from build123d import *

# Parameters (mm, degrees)
EXTRUDE_4_DEPTH     = 45
SKETCH_2_R          = 2.5
CUT_EXTRUDE_1_DEPTH = 85.798913103


with BuildPart() as part:
    # 草图1 → 凸台-拉伸4 (new body)
    with BuildSketch(Plane.XY):
        with BuildLine():
            ThreePointArc((11.999755772, 64.190702015), (7.19287537, 69.699227744), (0.441332655, 66.894477154))
            Line((0.441332655, 66.894477154), (-16.87917542, 36.894477154))
            Line((-16.87917542, 36.894477154), (-16.87917542, -3.105522846))
            Line((-16.87917542, -3.105522846), (-5.332170037, -23.105522846))
            Line((-5.332170037, -23.105522846), (9.992741519, -33.105522846))
            Line((9.992741519, -33.105522846), (11.999755772, -30.029791253))
            Line((11.999755772, -30.029791253), (-6.87917542, -3.105522846))
            Line((-6.87917542, -3.105522846), (-6.87917542, 14.190702015))
            Line((-6.87917542, 14.190702015), (-6.87917542, 24.190702015))
            Line((-6.87917542, 24.190702015), (10.114332844, 34.190702015))
            Line((10.114332844, 34.190702015), (11.999755772, 64.190702015))
        make_face()
    extrude(amount=EXTRUDE_4_DEPTH)

    # 草图2 → 切除-拉伸1 (cut, through all)
    with BuildSketch(Plane.XY):
        with Locations(Location((5.784422652, 63.881230161, 0), (0, 0, 180))):
            Circle(SKETCH_2_R)
    extrude(amount=CUT_EXTRUDE_1_DEPTH, mode=Mode.SUBTRACT)


solid = part.part
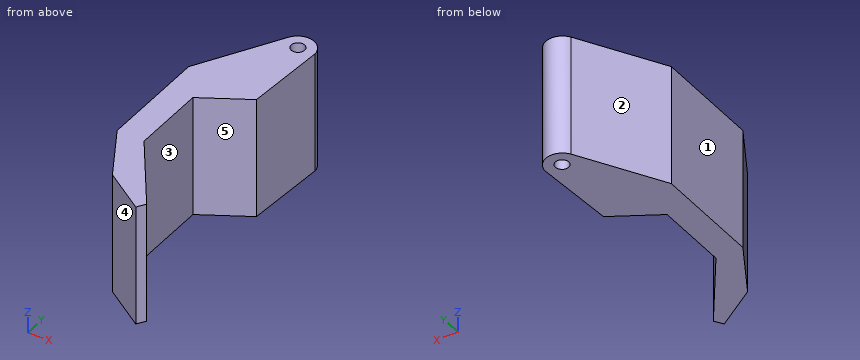
Can you work these out from the model? Positions are in its coordinate system, mm. Face numbers are marked on the shaded views. A direction names the side the tool comes from. Round coordinates to 2 decimals unless told otherwise and drop trailing zeros. Loops run counter-clockwise (first coordinate to the right, second up) from the corner with the lowest first, then second, coordinate; pieces in that order, holes last. Notation, with made-up numbers: (54.25, -5.5) - (70.25, -5.5) arc R21 cw to (70.25, 11.5) - close; hole circle Ø8 at (82.25, 22). An arc over 180 degrees is marked (long way). Use CSV: the item, a comma, the result in double quotes. Start each with the question number.
1) If we section it at C-C on x = -4: Write out the boundary of the cut face in (y, z).
2) For pin 1 Ø1 at (x, z) = (-5, 27.5) entering from +Y; pin 2 Ø4.5 at (x, y) = (5.78, 63.88) entering from +Z; pin 3 Ø12 at (x, z) = (1.5, 23.5) entering from -Y; pin 4 Ø5 at (x, z) = (-3.5, 29) entering from +Y, each with a flat end and sliding along its axis, tell me the tip position at first contact or that it passes through.
3) If we section it at B-B on z = 4.5: Write out the boundary of the cut face in (x, y), plus the area to 3 significant figures.
4) If we section it at A-A on x = 5.75: Write out the boundary of the cut face in (y, z).
5) For the marked faces 4 and 5, which set-ups out of +Z, -Z, +X, -X, +Y, -Y let a thin tool reach every point of the face, with its end or its side?
6) Please list where these lines run through material, in increasing order: probe 1 along Y at (x, z) = (6.5, 32); probe 2 along X at (y, z) = (3, 6); probe 3 along X at (y, z) = (63.5, 3). Write a range as [from, to].
7) If we section it at D-D on y = 17: Write out the boundary of the cut face in (x, z), plus the area to 3 significant figures.
8) We'd pull the mould along Y, two halves only. Please class the marked faces 1, 2 and 3: released by +Y, released by -Y, zero draft, split by the parting line, or undercut.
Geometry results:
1,outline,"(-23.97, 0) - (-7.21, 0) - (-7.21, 45) - (-23.97, 45) - close; (25.88, 0) - (59.2, 0) - (59.2, 45) - (25.88, 45) - close"
2,pin 1,"stops at y = 58.34"
2,pin 2,"passes through"
2,pin 3,"stops at y = -31.48"
2,pin 4,"stops at y = 64.4"
3,outline,"(-16.88, -3.11) - (-5.33, -23.11) - (9.99, -33.11) - (12, -30.03) - (-6.88, -3.11) - (-6.88, 24.19) - (10.11, 34.19) - (12, 64.19) arc R6.26 ccw to (0.44, 66.89) - (-16.88, 36.89) - close; hole circle Ø5 at (5.78, 63.88)"
3,area,"1,420 mm2"
4,outline,"(-30.34, 0) - (-21.12, 0) - (-21.12, 45) - (-30.34, 45) - close; (31.62, 0) - (61.38, 0) - (61.38, 45) - (31.62, 45) - close; (66.38, 0) - (69.86, 0) - (69.86, 45) - (66.38, 45) - close"
5,face 4,"+Z, -Z, -X, -Y"
5,face 5,"+Z, -Z, +X"
6,probe 1,"y = [-30.83, -22.19], [32.06, 61.49], [66.28, 69.82]"
6,probe 2,"x = [-16.88, -6.88]"
6,probe 3,"x = [-1.52, 3.31], [8.26, 11.96]"
7,outline,"(-16.88, 0) - (-6.88, 0) - (-6.88, 45) - (-16.88, 45) - close"
7,area,"450 mm2"
8,face 1,"zero draft"
8,face 2,"released by +Y"
8,face 3,"undercut"
